Input: part model. Units: mm. Frame: model coordinates. Face numbers are marked on the shaded views. A direction names the side the tool comes from. Round coordinates to 2 decimals unless told otherwise and drop trailing zeros. Order: outer loops, then holes, each group sorted by start corner. A loop starts at its lowest first (then second) coordinate and runs counter-clockwise, first axis right, second up.
Item 1: Cut plane C-C on y = 39. Output: boundary loops of the cut face in (x, z), then the cut area to 3 significant figures.
Item 2: Line query: L1, parallel to Y at x = 15, z = 8.8; L2, parallel to Y at x = 25, z = 13; L3, parallel to Z at x = 18, y = -15.5. Output: solid intervals per line, ascending.
Item 3: Cut plane A-A on y = 30. Output: boundary loops of the cut face in (x, z), then the cut area to 3 significant figures.
Item 4: Mould query, pull axis Y, two halves, no side actions, for the marked faces 5, 6 and 7. Classes: released by +Y, released by -Y, zero draft, split by the parting line, or undercut.
Item 5: Reachability of the marked faces 1, 2, 3 and 4 from +Z, -Z, +X, -X, +Y, -Y: full face, straight path, thin tool, end or side. Return the list, or none.
Item 6: Cut plane B-B on z = 19.5. Give the number of separate pieces and of enclosed holes in the cut face, then the cut area to 3 significant figures.
Item 7: First-contact query: pin 1 (10 mm diameter, centred on x = 22.5, y = -4.5, fed in from +Z); pin 2 (11.5 mm diameter, centred on x = 15.5, y = 31, fed in from +Z); pin 3 (10 mm diameter, centred on x = 14, y = 3, fed in from +Z); pin 4 (8 mm diameter, centred on y = 17.5, z = 18, fed in from +X). Flat tips, straight axial feed; report the tip coordinate or a pass-through.
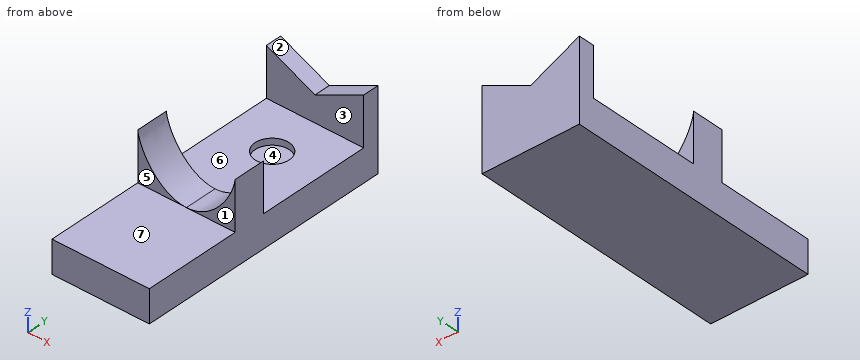
Autodesk Inventor part; units mm, degrees
ref_plane "YZ Plane" through (0, 0, 0) normal (1, 0, 0) x (0, 1, 0)
ref_plane "XZ Plane" through (0, 0, 0) normal (0, 1, 0) x (-1, 0, 0)
ref_plane "XY Plane" through (0, 0, 0) normal (0, 0, 1) x (1, 0, 0)
sketch "Sketch1" plane through (0, 0, 0) normal (0, 0, 1) x (1, 0, 0)
  line L0 (0, 0) -> (30, 0)
  line L1 (30, 0) -> (30, -30)
  line L2 (30, -30) -> (0, -30)
  line L3 (0, -30) -> (0, 0)
  dimension "d2" = 30
  dimension "d3" = 30
extrude "Extrusion1" add sketch "Sketch1" along normal blind 10
sketch "Sketch2" plane through (0, 0, 0) normal (0, 1, 0) x (1, 0, 0)
  line L0 (30, -10) -> (0, -10)
  line L1 (30, -10) -> (30, -25)
  line L2 (0, 0) -> (0, -10)
  line L3 (0, -25) -> (0, -10)
  spline S0 degree 4 poles (30, -25) (29.1667, -16.6667) (15, 3.8889) (0.8333, -16.6667) (0, -25) knots 0 0 0 0 0 1 1 1 1 1
  line L4 (15, -10) -> (30, -10) construction
  line L5 (15, -10) -> (0, -10) construction
  line L6 (0, -10) -> (5, -15) construction
  line L7 (5, -15) -> (25, -15) construction
  line L8 (30, -10) -> (25, -15) construction
  point P0 (24.1347, -10)
  point P1 (8.1347, -10)
  point P2 (15, -10)
  point P3 (0, -25)
  point P4 (30, -25)
  dimension "d16" = 15
  dimension "d18" = 0
  dimension "d19" = 5
  dimension "d20" = 5
extrude "Extrusion2" add sketch "Sketch2" along normal blind 10
sketch "Sketch3" plane through (0, 0, 0) normal (0, 1, 0) x (1, 0, 0)
  line L0 (0, 0) -> (30, 0)
  line L1 (0, 0) -> (0, -10)
  line L2 (30, 0) -> (30, -10)
  line L3 (15, -10) -> (0, -10)
  line L4 (30, -10) -> (15, -10)
extrude "Extrusion3" add sketch "Sketch3" along normal blind 50
sketch "Sketch4" plane through (0, 50, 0) normal (0, 1, 0) x (1, 0, 0)
  line L0 (30, -10) -> (30, -25)
  line L1 (30, -25) -> (15, -18)
  line L2 (15, -18) -> (0, -25)
  line L3 (0, -25) -> (0, -10)
  line L4 (0, -10) -> (30, -10)
  line L5 (30, -10) -> (0, -10)
  dimension "d27" = 8
  dimension "d28" = 15
extrude "Extrusion4" add sketch "Sketch4" against normal blind 5
sketch "Sketch5" plane through (0, 10, 10) normal (0, 0, 1) x (1, 0, 0)
  circle A0 centre (15, 20) radius 5.25
  line L0 (15, 20) -> (30, 20) construction
  line L1 (15, 20) -> (0, 20) construction
  line L2 (30, 0) -> (30, 35) construction
  line L3 (0, 0) -> (0, 35) construction
  line L4 (15, 0) -> (0, 0) construction
  point P0 (0, -10)
  point P1 (30, 40)
  point P2 (0, 40)
  dimension "d21" = 10.5
  dimension "d22" = 20
extrude "Extrusion5" cut sketch "Sketch5" against normal blind 2
properties part number "stand"
From the geometry:
1. outline: (0, 0) - (30, 0) - (30, 10) - (0, 10) - close
1. area: 300 mm2
2. L1: y = -30 to 24.75, 35.25 to 50
2. L2: y = 0 to 10, 45 to 50
2. L3: z = 0 to 10
3. outline: (0, 0) - (30, 0) - (30, 10) - (20.25, 10) - (20.25, 8) - (9.75, 8) - (9.75, 10) - (0, 10) - close
3. area: 279 mm2
4. face 5: released by -Y
4. face 6: undercut
4. face 7: zero draft
5. face 1: +Z, +X, -X, -Y
5. face 2: +Z, +Y, -Y
5. face 3: +Z, +X, -X
5. face 4: +Z
6. separate pieces: 4
6. enclosed holes: 0
6. area: 155 mm2
7. pin 1: stops at z = 14.66
7. pin 2: stops at z = 10
7. pin 3: stops at z = 11.7
7. pin 4: passes through
